```python
from build123d import *

# Parameters (mm, degrees)
SKETCH1_R           = 1.1
BOSS_EXTRUDE1_DEPTH = 7.8


with BuildPart() as part:
    # Sketch1 → Boss-Extrude1 (new body)
    # profile 1 of 5: a face of its own
    with BuildSketch(Plane(origin=(0, 0, 0), x_dir=(1, 0, 0), z_dir=(0, 1, 0))):
        with BuildLine():
            ThreePointArc((-1.5, -0.901387819), (-0.861705088, -1.523142916), (0, -1.75))
            ThreePointArc((0, -1.75), (0.861705088, -1.523142916), (1.5, -0.901387819))
            Line((1.5, -0.901387819), (1.5, 0.901387819))
            ThreePointArc((1.5, 0.901387819), (0.861705088, 1.523142916), (0, 1.75))
            ThreePointArc((0, 1.75), (-0.861705088, 1.523142916), (-1.5, 0.901387819))
            Line((-1.5, 0.901387819), (-1.5, -0.901387819))
        make_face()
        with Locations(Location((0, 0, 0), (0, 0, 270))):
            Circle(SKETCH1_R, mode=Mode.SUBTRACT)
    # profile 2 of 5: a face of its own
    with BuildSketch(Plane(origin=(0, 0, 0), x_dir=(1, 0, 0), z_dir=(0, 1, 0))):
        with BuildLine():
            ThreePointArc((-1.5, 0.901387819), (-1.75, 0), (-1.5, -0.901387819))
            Line((-1.5, -0.901387819), (-1.5, 0.901387819))
        make_face()
    # profile 3 of 5: a face of its own
    with BuildSketch(Plane(origin=(0, 0, 0), x_dir=(1, 0, 0), z_dir=(0, 1, 0))):
        with BuildLine():
            Line((1.5, 0.901387819), (1.5, -0.901387819))
            ThreePointArc((1.5, -0.901387819), (1.686342195, -0.467707173), (1.75, 0))
            ThreePointArc((1.75, 0), (1.686342195, 0.467707173), (1.5, 0.901387819))
        make_face()
    # profile 4 of 5: a face of its own
    with BuildSketch(Plane(origin=(0, 0, 0), x_dir=(1, 0, 0), z_dir=(0, 1, 0))):
        with BuildLine():
            Line((0, -1.75), (1.5, -1.75))
            Line((1.5, -1.75), (1.5, -0.901387819))
            ThreePointArc((1.5, -0.901387819), (0.861705088, -1.523142916), (0, -1.75))
        make_face()
    # profile 5 of 5: a face of its own
    with BuildSketch(Plane(origin=(0, 0, 0), x_dir=(1, 0, 0), z_dir=(0, 1, 0))):
        with BuildLine():
            Line((-1.5, -1.75), (0, -1.75))
            ThreePointArc((0, -1.75), (-0.861705088, -1.523142916), (-1.5, -0.901387819))
            Line((-1.5, -0.901387819), (-1.5, -1.75))
        make_face()
    extrude(amount=BOSS_EXTRUDE1_DEPTH)


solid = part.part
```
Part model, mm, in its own coordinate system. A direction names the side the tool comes from. Round coordinates to 2 decimals unless told otherwise and drop trailing zeros. Loops run counter-clockwise (first coordinate to the right, second up) from the corner with the lowest first, then second, coordinate; pieces in that order, holes last. Notation, with made-up numbers: (44.5, 81.5) -> (75.5, 81.5) arc R10 cw to (75.5, 99.5) -> close; hole circle Ø4 at (31.5, 6). An arc over 180 degrees is marked (long way). Use one line per item in the form item = value. Start each with the question number.
Item 1: Band-saw the part on B-B (z = 0.45). List the corners of the cut face in (x, y), plus the area to 3 significant figures.
Item 2: Drop flat-ended pins along their axis: pin 1 Ø0.9 at (y, z) = (6, 1.5) entering from -X; pin 2 Ø1.8 at (x, z) = (0, 0) entering from -Y. Give the stop position or say it passes through.
Item 3: Drill centre lines: line 1 along Z through (x, y) = (-0.05, 3.75); line 2 along Z through (x, y) = (0.4, 3); line 3 along X through (y, z) = (6, 0.6). Where is each one in solid material? Low to high.
Item 4: Two-plate mould, pull along Z, no slides. Class faces 1 (the cylindrical face through (1.09, 3.85, -0.14)), 2 (the flat face through (-1, 0, 1)), 3 (the flat face through (0, 4, 1.75)): released by +Z, released by -Z, zero draft, split by the parting line, or undercut.
Item 5: Band-saw the part on A-A (y = 5.25). List the corners of the cut face in (x, z), plus the area to 3 significant figures.
Item 6: Tool access for faces 4 (the flat face through (1.5, 3.8, 1.3)), 5 (the flat face through (-1, 7.8, 1)), 6 (the flat face through (-1.5, 3.8, 1.3)): list every direction of +Z, -Z, +X, -X, +Y, -Y with a clear straight run to the whole face (end or side of a thin tool).
Item 7: Band-saw the part on C-C (x = -0.25). List the corners of the cut face in (y, z).
Data:
q1.outline = (-1.69, 0) -> (-1, 0) -> (-1, 7.8) -> (-1.69, 7.8) -> close; (1, 0) -> (1.69, 0) -> (1.69, 7.8) -> (1, 7.8) -> close
q1.area = 10.7 mm^2
q2.pin_1 = -1.5
q2.pin_2 = through
q3.line_1 = -1.75 to -1.1, 1.1 to 1.75
q3.line_2 = -1.7 to -1.02, 1.02 to 1.75
q3.line_3 = -1.64 to -0.92, 0.92 to 1.64
q4.face_1 = undercut
q4.face_2 = zero draft
q4.face_3 = released by +Z
q5.outline = (-1.5, 0.9) arc R1.75 ccw (long way) to (1.5, 0.9) -> (1.5, 1.75) -> (-1.5, 1.75) -> close; hole circle Ø2.2 at (0, 0)
q5.area = 6.56 mm^2
q6.face_4 = +Z, +X, +Y, -Y
q6.face_5 = +Z, -Z, +X, -X, +Y
q6.face_6 = +Z, -X, +Y, -Y
q7.outline = (0, -1.73) -> (7.8, -1.73) -> (7.8, -1.07) -> (0, -1.07) -> close; (0, 1.07) -> (7.8, 1.07) -> (7.8, 1.75) -> (0, 1.75) -> close
